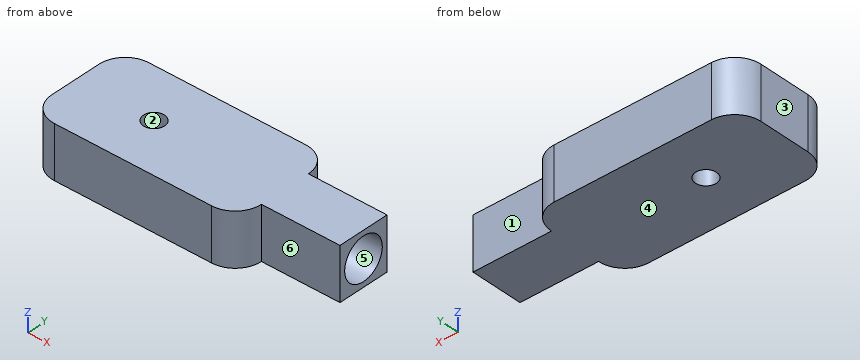
from build123d import *

# Parameters (mm, degrees)
SKETCH2_W           = 50.8
SKETCH2_H           = 25.4
BOSS_EXTRUDE1_DEPTH = 12.7
FILLET1_R           = 6.35
SKETCH3_R           = 2.54
CUT_EXTRUDE1_DEPTH  = 32.108519733
SKETCH4_W           = 12.7
SKETCH4_H           = 12.7
BOSS_EXTRUDE2_DEPTH = 19.05
SKETCH5_R           = 5.08
CUT_EXTRUDE2_DEPTH  = 25.4


with BuildPart() as part:
    # Sketch2 → Boss-Extrude1 (new body)
    with BuildSketch(Plane.XY):
        Rectangle(SKETCH2_W, SKETCH2_H)
    extrude(amount=BOSS_EXTRUDE1_DEPTH)

    # Fillet1
    fillet1_edges = [part.edges().sort_by_distance(p)[0] for p in [
        (-25.4, 12.7, 6.35),
        (25.4, 12.7, 6.35),
        (25.4, -12.7, 6.35),
        (-25.4, -12.7, 6.35),
    ]]
    fillet(fillet1_edges, radius=FILLET1_R)

    # Sketch3 → Cut-Extrude1 (cut, through all)
    with BuildSketch(Plane.XY.offset(12.7)):
        with Locations((-6.35, 0)):
            Circle(SKETCH3_R)
    extrude(amount=-CUT_EXTRUDE1_DEPTH, mode=Mode.SUBTRACT)

    # Sketch4 → Boss-Extrude2 (add)
    with BuildSketch(Plane(origin=(25.4, 0, 0), x_dir=(0, 0, -1), z_dir=(1, 0, 0))):
        with Locations((-6.35, 0)):
            Rectangle(SKETCH4_W, SKETCH4_H)
    extrude(amount=BOSS_EXTRUDE2_DEPTH)

    # Sketch5 → Cut-Extrude2 (cut)
    with BuildSketch(Plane(origin=(44.45, 0, 0), x_dir=(0, 0, -1), z_dir=(1, 0, 0))):
        with Locations((-6.35, 0)):
            Circle(SKETCH5_R)
    extrude(amount=-CUT_EXTRUDE2_DEPTH, mode=Mode.SUBTRACT)


solid = part.part
Could you check a few things on this model? Use its own coordinates, in mm. Face numbers are marked on the shaded views. A direction names the side the tool comes from. Round coordinates to 2 decimals unless told otherwise and drop trailing zeros. Order: outer loops, then holes, each group sorted by start corner. A loop starts at its lowest first (then second) coordinate and runs counter-clockwise, first axis right, second up.
(1) Please list where these lines run through material, in increasing order: line 1 along Y through (x, z) = (-6.35, 5.5); line 2 along Z through (x, y) = (35, -2.5); line 3 along X through (y, z) = (2.25, 5.5).
Response values:
line 1: y = -12.7 to -2.54, 2.54 to 12.7
line 2: z = 0 to 1.93, 10.77 to 12.7
line 3: x = -25.4 to -7.53, -5.17 to 19.05
(2) Imagine slicing it at D-D (x = 21). Write out the boundary of the cut face in (y, z), plus the area to 3 significant figures.
Response values:
outline: (-12.39, 0) - (12.39, 0) - (12.39, 12.7) - (-12.39, 12.7) - close; hole circle Ø10.16 at (0, 6.35)
area: 234 mm2
(3) Which directions (+Z, -Z, +X, -X, +Y, -Y) give clear straight access to the entire face, cutting with the end or side of a thin tool? Please do the marked faces 4, 5 and 6.
Response values:
face 4: -Z, +X, -X, +Y, -Y
face 5: +X
face 6: +Z, -Z, +X, -Y
(4) I'm going to push flat-ended pins straight in: pin 1 (5 mm diameter, centred on y = -9, z = 2.5, fed in from -X); pin 2 (1.5 mm diameter, centred on y = -10, z = 5, fed in from +X). Where does each tip first touch, or does it pass through?
Response values:
pin 1: stops at x = -25.4
pin 2: stops at x = 24.7
(5) If we mould it in two halves opening along X, with no side actions, what happens to the marked faces 1, 2 and 3? For each: released by +X, released by -X, zero draft, split by the parting line, or undercut.
Response values:
face 1: zero draft
face 2: undercut
face 3: released by -X
(6) Imagine slicing it at B-B (y = 0). Write out the boundary of the cut face in (x, z), plus the area to 3 significant figures.
Response values:
outline: (-25.4, 0) - (-8.89, 0) - (-8.89, 12.7) - (-25.4, 12.7) - close; (-3.81, 0) - (44.45, 0) - (44.45, 1.27) - (19.05, 1.27) - (19.05, 11.43) - (44.45, 11.43) - (44.45, 12.7) - (-3.81, 12.7) - close
area: 565 mm2
(7) Imagine slicing it at A-A (x = -6.35). Write out the boundary of the cut face in (y, z).
Response values:
outline: (-12.7, 0) - (-2.54, 0) - (-2.54, 12.7) - (-12.7, 12.7) - close; (2.54, 0) - (12.7, 0) - (12.7, 12.7) - (2.54, 12.7) - close
